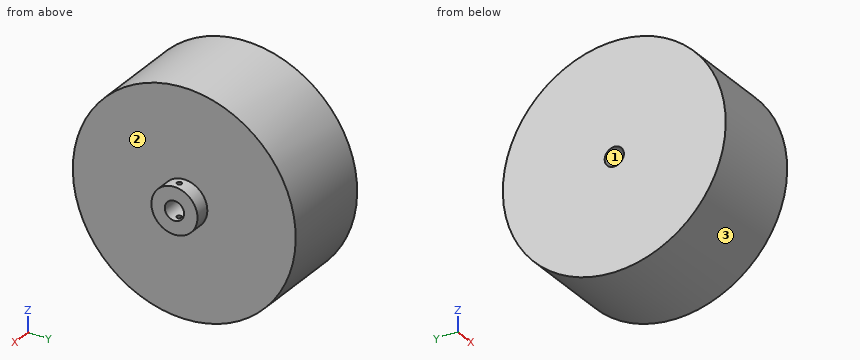
```python
from build123d import *

# Parameters (mm, degrees)
SKETCH1_R               = 36.83
BOSS_EXTRUDE1_DEPTH     = 31.75
SKETCH3_R               = 7.62
BOSS_EXTRUDE2_DEPTH     = 5.08
BOSS_EXTRUDE3_START     = -31.75
SKETCH3_2_R             = 7.62
BOSS_EXTRUDE3_DEPTH     = 5.08
SKETCH2_R               = 3.175
CUT_EXTRUDE1_DEPTH      = 6.08
CUT_EXTRUDE1_DEPTH_BACK = 37.83
SKETCH4_R               = 0.79375
CUT_EXTRUDE2_DEPTH      = 37.83
CUT_EXTRUDE2_DEPTH_BACK = 37.83
SKETCH5_W               = 11.37457975
SKETCH5_H               = 27.007523476
CUT_EXTRUDE3_DEPTH      = 37.83
CUT_EXTRUDE3_DEPTH_BACK = 37.83


with BuildPart() as part:
    # Sketch1 → Boss-Extrude1 (new body)
    with BuildSketch(Plane(origin=(0, 0, 0), x_dir=(0, 0, -1), z_dir=(1, 0, 0))):
        Circle(SKETCH1_R)
    extrude(amount=BOSS_EXTRUDE1_DEPTH)

    # Sketch3 → Boss-Extrude2 (add)
    with BuildSketch(Plane(origin=(31.75, 0, 0), x_dir=(0, 0, -1), z_dir=(1, 0, 0))):
        Circle(SKETCH3_R)
    extrude(amount=BOSS_EXTRUDE2_DEPTH)

    # Sketch3<2> → Boss-Extrude3 (add)
    with BuildSketch(Plane(origin=(31.75, 0, 0), x_dir=(0, 0, -1), z_dir=(1, 0, 0)).offset(BOSS_EXTRUDE3_START)):
        Circle(SKETCH3_2_R)
    extrude(amount=-BOSS_EXTRUDE3_DEPTH)

    # Sketch2 → Cut-Extrude1 (cut, two sides)
    with BuildSketch(Plane(origin=(31.75, 0, 0), x_dir=(0, 0, -1), z_dir=(1, 0, 0))) as cut_extrude1_sk:
        Circle(SKETCH2_R)
    extrude(amount=CUT_EXTRUDE1_DEPTH, mode=Mode.SUBTRACT)
    extrude(cut_extrude1_sk.sketch, amount=-CUT_EXTRUDE1_DEPTH_BACK, mode=Mode.SUBTRACT)

    # Sketch4 → Cut-Extrude2 (cut, two sides)
    with BuildSketch(Plane.XY) as cut_extrude2_sk:
        with Locations((34.29, 0)):
            Circle(SKETCH4_R)
        with Locations((-2.54, 0)):
            Circle(SKETCH4_R)
    extrude(amount=CUT_EXTRUDE2_DEPTH, mode=Mode.SUBTRACT)
    extrude(cut_extrude2_sk.sketch, amount=-CUT_EXTRUDE2_DEPTH_BACK, mode=Mode.SUBTRACT)

    # Sketch5 → Cut-Extrude3 (cut, two sides)
    with BuildSketch(Plane(origin=(0, 0, 0), x_dir=(1, 0, 0), z_dir=(0, 1, 0))) as cut_extrude3_sk:
        with Locations((-5.687289875, -0.244411977)):
            Rectangle(SKETCH5_W, SKETCH5_H)
    extrude(amount=CUT_EXTRUDE3_DEPTH, mode=Mode.SUBTRACT)
    extrude(cut_extrude3_sk.sketch, amount=-CUT_EXTRUDE3_DEPTH_BACK, mode=Mode.SUBTRACT)


solid = part.part
```
Source: CAD feature listing. Evaluate the final solid. Frame: model axes, mm. Face numbers are marked on the shaded views. Round coordinates to 2 decimals unless told otherwise and drop trailing zeros. Loops run counter-clockwise (first coordinate to the right, second up) from the corner with the lowest first, then second, coordinate; pieces in that order, holes last. Notation, with made-up numbers: M 4.5,77.5 L 12.5,77.5 A30 cw 12.5,101.5 Z; hole C -28.75,68 d7. An arc over 180 degrees is marked long. Use a Markdown table: item, result. Add a question column.
1. Pull-direction query (Z, two-part tool) for the marked faces 1, 2 and 3; classes: +Z half, -Z half, draft (parallel to the pull), parting line (faces both ways), or undercut.
2. Ray query, line 1 along Y through (x, z) = (25, 0) (3 decimals); line 2 along Y through (x, z) = (34, 5); line 3 along X through (y, z) = (24, -12). Return the intervals inside material, ascending. Write a range as [from, to].
3. Cut plane A-A, the plane z = 0. Output: boundary loops of the cut face in (x, y) (3 decimals), and give its area (3 significant figures).
4. Contact query for flat-ended pins moving along their axis: pin 1 (1.8 mm diameter, centred on x = 34.29, y = 0, fed in from -Z); pin 2 (4 mm diameter, centred on x = 16.5, y = 20, fed in from -Z); pin 3 (1.5 mm diameter, centred on x = 30.5, z = 6, fed in from +Y); pin 4 (10 mm diameter, centred on y = 13, z = -9, fed in from -X). Output: stop coordinate, or through.
5. Cut plane D-D, the plane z = 9.5. Output: boundary loops of the cut face in (x, y).
6. Cut plane B-B, the plane x = 16. Output: boundary loops of the cut face in (y, z) (3 decimals), and give its area (3 significant figures).
7. Cut plane C-C, the plane y = 26.5. Output: boundary loops of the cut face in (x, z).
Solution:
| question | item | result |
|---|---|---|
| 1 | face 1 | undercut |
| 1 | face 2 | draft |
| 1 | face 3 | parting line |
| 2 | line 1 | y = [-36.83, -3.175], [3.175, 36.83] |
| 2 | line 2 | y = [-5.75, -0.74], [0.74, 5.75] |
| 2 | line 3 | x = [0, 31.75] |
| 3 | outline | M 0,-36.83 L 31.75,-36.83 L 31.75,-7.62 L 36.83,-7.62 L 36.83,-3.175 L 0,-3.175 Z; M 0,3.175 L 36.83,3.175 L 36.83,7.62 L 31.75,7.62 L 31.75,36.83 L 0,36.83 Z |
| 3 | area | 2,180 mm2 |
| 4 | pin 1 | stops at z = -7.62 |
| 4 | pin 2 | stops at z = -32.13 |
| 4 | pin 3 | stops at y = 36.45 |
| 4 | pin 4 | stops at x = 0 |
| 5 | outline | M 0,-35.58 L 31.75,-35.58 L 31.75,35.58 L 0,35.58 Z |
| 6 | outline | C 0,0 d73.66; hole C 0,0 d6.35 |
| 6 | area | 4,230 mm2 |
| 7 | outline | M 0,-25.58 L 31.75,-25.58 L 31.75,25.58 L 0,25.58 Z |
